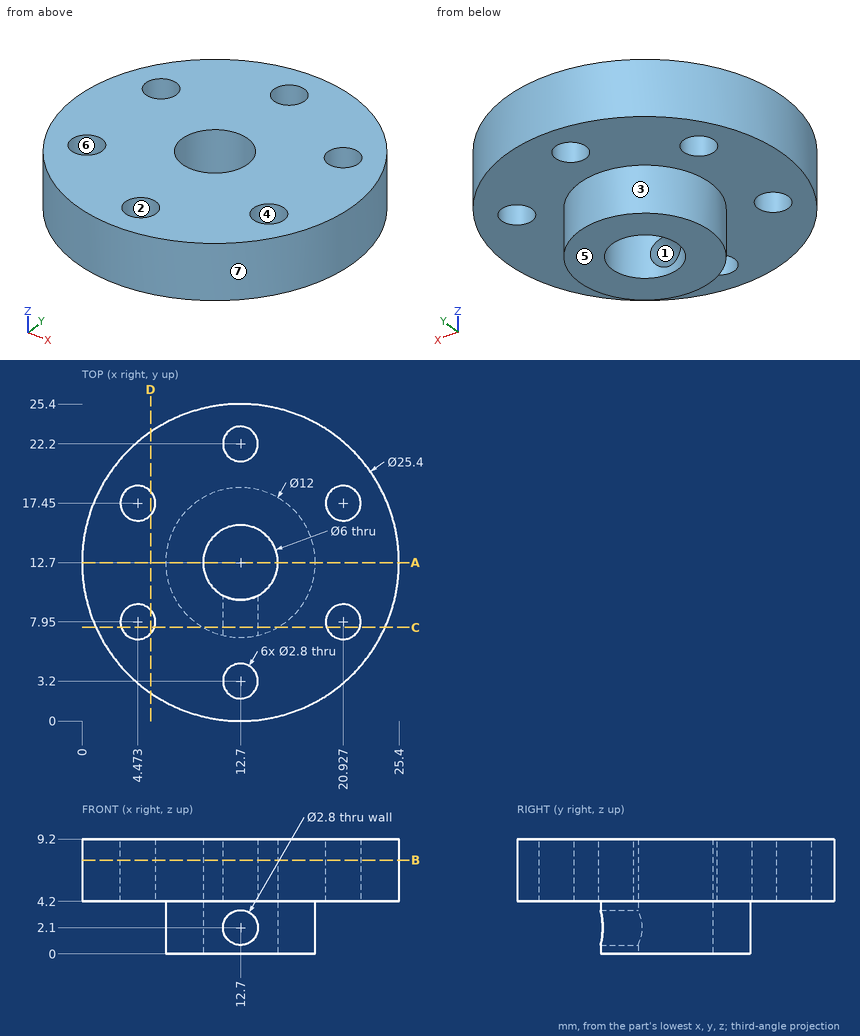
Study the drawing (mm; zero at the part's minimum x, y, z) and answer. A direction names the side the tool comes from. Round coordinates to 2 decimals unless told otherwise and drop trailing zeros. Loops run counter-clockwise (first coordinate to the right, second up) from the corner with the lowest first, then second, coordinate; pieces in that order, holes last. Notation, with made-up numbers: (11.25, 6.25) -> (59.25, 6.25) arc R20 cw to (59.25, 43.25) -> close; hole circle Ø2 at (57, -8). An arc over 180 degrees is marked (long way). Write each question's results on one line, items separated by ' | '. Start each with the question number.
1. For a pull along X with two mould halves and no side action, classify the marked faces 4, 5, 6 and 7 as +X half, -X half, draft (parallel to the pull), parting line (faces both ways), or undercut.
2. A tool of negligible diameter and unlimited length cuts with its end or side. For the marked faces 1, 2 and 3, from which of +Z, -Z, +X, -X, +Y, -Y can it reach the whole face along a straight path? Write none if from no direction.
3. Section A-A (y = 12.7) is taken. Determine the outline of the cut face in (x, z), plus the area to 3 significant figures.
4. Find the intervals of material crossed by probe 1 along Z at (x, y) = (12.7, 8.85); probe 2 along Z at (x, y) = (13.5, 8.25); probe 3 along Z at (x, y) = (17, 3.5), in increasing order. Write a range as from..to.
5. Section C-C (y = 7.5) is taken. Determine the outline of the cut face in (x, z), plus the area to 3 significant figures.
6. Section B-B (z = 7.5) is taken. Determine the outline of the cut face in (x, y).
7. Given pin 1 Ø1 at (y, z) = (15.5, 4.5) entering from +X; pin 2 Ø2 at (x, z) = (12.7, 2.1) entering from +Y; pin 3 Ø4.5 at (x, y) = (12.7, 22.2) entering from -Z, each flat-ended and moving along its own axis, determine where each tip first touches the part or whether it passes through.
8. Section D-D (x = 5.5) is taken. Determine the outline of the cut face in (y, z), plus the area to 3 significant figures.
Evaluation:
1) face 4: undercut | face 5: draft | face 6: undercut | face 7: parting line
2) face 1: -Y | face 2: +Z, -Z | face 3: -Z
3) outline: (0, 4.2) -> (6.7, 4.2) -> (6.7, 0) -> (9.7, 0) -> (9.7, 9.2) -> (0, 9.2) -> close; (15.7, 0) -> (18.7, 0) -> (18.7, 4.2) -> (25.4, 4.2) -> (25.4, 9.2) -> (15.7, 9.2) -> close | area: 122 mm2
4) probe 1: z = 0..0.7, 3.5..9.2 | probe 2: z = 0..0.95, 3.25..9.2 | probe 3: z = 4.2..9.2
5) outline: (1.11, 4.2) -> (3.15, 4.2) -> (3.15, 9.2) -> (1.11, 9.2) -> close; (5.8, 4.2) -> (9.71, 4.2) -> (9.71, 0) -> (15.69, 0) -> (15.69, 4.2) -> (19.6, 4.2) -> (19.6, 9.2) -> (5.8, 9.2) -> close; (22.25, 4.2) -> (24.29, 4.2) -> (24.29, 9.2) -> (22.25, 9.2) -> close; hole circle Ø2.8 at (12.7, 2.1) | area: 108 mm2
6) outline: circle Ø25.4 at (12.7, 12.7); hole circle Ø2.8 at (4.47, 7.95); hole circle Ø2.8 at (4.47, 17.45); hole circle Ø6 at (12.7, 12.7); hole circle Ø2.8 at (12.7, 3.2); hole circle Ø2.8 at (12.7, 22.2); hole circle Ø2.8 at (20.93, 7.95); hole circle Ø2.8 at (20.93, 17.45)
7) pin 1: stops at x = 25.19 | pin 2: stops at y = 18.7 | pin 3: stops at z = 4.2
8) outline: (2.24, 4.2) -> (7, 4.2) -> (7, 9.2) -> (2.24, 9.2) -> close; (8.9, 4.2) -> (16.5, 4.2) -> (16.5, 9.2) -> (8.9, 9.2) -> close; (18.4, 4.2) -> (23.16, 4.2) -> (23.16, 9.2) -> (18.4, 9.2) -> close | area: 85.6 mm2
